from build123d import *

# Parameters (mm, degrees)
F0_W     = 40.4
F0_H     = 19.8
F1_DEPTH = 36
F2_SIZE  = 5.5
F3_R     = 7
F3_R_2   = 5
F4_DEPTH = 3
F5_DEPTH = 3
F6_SIZE  = 2.99999
F7_R     = 3
F8_DEPTH = 4


# Not quite as in the source:
# - a fillet or chamfer is up to 0.001 mm smaller than in the source, because OpenCascade refuses the exact size


with BuildPart() as f1:
    # F0 (on Top) → F1 (new body)
    with BuildSketch(Plane.XY):
        with Locations((0.6492929533, -3.5976961023)):
            Rectangle(F0_W, F0_H)
    extrude(amount=F1_DEPTH)

    # F2
    f2_edges = [f1.edges().sort_by_distance(p)[0] for p in [
        (-19.550707, -3.597696, 36),
    ]]
    chamfer(f2_edges, length=F2_SIZE)

    # F3 (on face) → F4 (join)
    with BuildSketch(Plane.XY.offset(36)):
        with Locations((10.8492929533, -3.5976961023)):
            Circle(F3_R)
        with Locations((10.8492929533, -3.5976961023)):
            Circle(F3_R_2, mode=Mode.SUBTRACT)
    extrude(amount=F4_DEPTH)

    # F5 (add): a face of the model
    f5_faces = [f1.faces().sort_by_distance(p)[0] for p in [
        (10.8492929533, -3.5976961023, 36),
    ]]
    extrude(f5_faces, amount=F5_DEPTH)

    # F6 (size 3 in the source; OpenCascade refuses exactly that, so slightly less here)
    f6_edges = [f1.edges().sort_by_distance(p)[0] for p in [
        (3.849293, -3.597696, 39),
    ]]
    chamfer(f6_edges, length=F6_SIZE)

    # F7 (on face) → F8 (join)
    with BuildSketch(Plane.XY.offset(39)):
        with Locations((10.8492929533, -3.5976961023)):
            Circle(F7_R)
    extrude(amount=F8_DEPTH)


solid = f1.part
Geometry check sheet. Reference: the model listing, model coordinates, mm. A direction names the side the tool comes from. Round coordinates to 2 decimals unless told otherwise and drop trailing zeros. Loops run counter-clockwise (first coordinate to the right, second up) from the corner with the lowest first, then second, coordinate; pieces in that order, holes last. Notation, with made-up numbers: (-39, 17.25) - (14, 17.25) arc R22 ccw to (14, 35.25) - close; hole circle Ø8 at (-16.5, -32.5). An arc over 180 degrees is marked (long way). Answer as CSV lines item,"result".
(1) Cross-section at A-A, the plane y = 4.75. Enter the section's corners in (x, z).
Output values:
outline,"(-19.55, 0) - (20.85, 0) - (20.85, 36) - (-14.05, 36) - (-19.55, 30.5) - close"
(2) Cross-section at C-C, the plane z = 33. Enter the section's corners in (x, y), and give its area (3 significant figures).
Output values:
outline,"(-17.05, -13.5) - (20.85, -13.5) - (20.85, 6.3) - (-17.05, 6.3) - close"
area,"750 mm²"
(3) Set-up check for faces 1 (the face through (0, -3, 0)), 2 (the face through (13.71, -2.7, 40.97)): record each of +Z, -Z, +X, -X, +Y, -Y from which the full face is reachable in a straight line by a thin tool's end or side.
Output values:
face 1,"-Z, +X, -X, +Y, -Y"
face 2,"+Z"
(4) Material ranges on line 1 along Z through (x, y) = (-1, -1); line 2 along Z through (x, y) = (13.5, -8.25); line 3 along X through (y, z) = (-11.5, 32.5), recorded low to high.
Output values:
line 1,"z = 0 to 36"
line 2,"z = 0 to 37.65"
line 3,"x = -17.55 to 20.85"
(5) Cross-section at B-B, the plane x = -10. Enter the section's corners in (y, z).
Output values:
outline,"(-13.5, 0) - (6.3, 0) - (6.3, 36) - (-13.5, 36) - close"
(6) Depth check by flat-ended pin: pin 1 Ø10 at (x, y) = (-6, -5.5) entering from +Z; pin 2 Ø2 at (y, z) = (1.5, 35.5) entering from -X. Enter the tip coordinate at first touch or a pass-through.
Output values:
pin 1,"stops at z = 36"
pin 2,"stops at x = -15.55"
